from build123d import *

# Parameters (mm, degrees)
SKETCH_1_W          = 15
SKETCH_1_H          = 15
SKETCH_1_R          = 5.5
EXTRUDE_1_DEPTH     = 45
SKETCH_5_W          = 15
SKETCH_5_H          = 15
EXTRUDE_3_DEPTH     = 15
FILLET_2_R          = 7.5
SKETCH_6_R          = 2.1
CUT_EXTRUDE_1_DEPTH = 49.023431781
CUT_EXTRUDE_2_DEPTH = 8
SKETCH_9_W          = 8
SKETCH_9_H          = 8
SKETCH_9_R          = 1.6
EXTRUDE_4_DEPTH     = 7
FILLET_3_R          = 2
SKETCH_11_R         = 3.2
CUT_EXTRUDE_3_DEPTH = 3.75
SKETCH_12_R         = 1.7
CUT_EXTRUDE_4_DEPTH = 10


with BuildPart() as part:
    # ｽｹｯﾁ1 → ﾎﾞｽ - 押し出し1 (new body)
    with BuildSketch(Plane.XY):
        Rectangle(SKETCH_1_W, SKETCH_1_H)
        with Locations(Location((0, 0, 0), (0, 0, 180))):
            Circle(SKETCH_1_R, mode=Mode.SUBTRACT)
    extrude(amount=EXTRUDE_1_DEPTH)

    # ｽｹｯﾁ5 → ﾎﾞｽ - 押し出し3 (add)
    with BuildSketch(Plane.XY.offset(45)):
        Rectangle(SKETCH_5_W, SKETCH_5_H)
    extrude(amount=-EXTRUDE_3_DEPTH)

    # ﾌｨﾚｯﾄ2
    fillet_2_edges = [part.edges().sort_by_distance(p)[0] for p in [
        (0, -7.5, 45),
        (0, 7.5, 45),
    ]]
    fillet(fillet_2_edges, radius=FILLET_2_R - 0.0001)  # a hair under: the kernel refuses the full size

    # ｽｹｯﾁ6 → ｶｯﾄ - 押し出し1 (cut, through all)
    with BuildSketch(Plane(origin=(7.5, 0, 0), x_dir=(0, 0, -1), z_dir=(1, 0, 0))):
        with Locations((-37.5, 0)):
            Circle(SKETCH_6_R)
    extrude(amount=-CUT_EXTRUDE_1_DEPTH, mode=Mode.SUBTRACT)

    # ｽｹｯﾁ7 → ｶｯﾄ - 押し出し2 (cut)
    with BuildSketch(Plane(origin=(7.5, 0, 0), x_dir=(0, 0, -1), z_dir=(1, 0, 0))):
        with BuildLine():
            Line((-37.5, -9.5), (2, -9.5))
            Line((2, -9.5), (2, 9.5))
            Line((2, 9.5), (-37.5, 9.5))
            ThreePointArc((-37.5, 9.5), (-44.217514421, 6.717514421), (-47, 0))
            ThreePointArc((-47, 0), (-44.217514421, -6.717514421), (-37.5, -9.5))
        make_face()
    extrude(amount=-CUT_EXTRUDE_2_DEPTH, mode=Mode.SUBTRACT)

    # ｽｹｯﾁ9 → ﾎﾞｽ - 押し出し4 (add)
    # profile 1 of 4: a face of its own
    with BuildSketch(Plane(origin=(-0.5, 0, 0), x_dir=(0, 0, -1), z_dir=(1, 0, 0))):
        with Locations((-4, -9.477225575)):
            Rectangle(SKETCH_9_W, SKETCH_9_H)
        with Locations((-4, -9.477225575)):
            Circle(SKETCH_9_R, mode=Mode.SUBTRACT)
    # profile 2 of 4: a face of its own
    with BuildSketch(Plane(origin=(-0.5, 0, 0), x_dir=(0, 0, -1), z_dir=(1, 0, 0))):
        with Locations((-26, 9.477225575)):
            Rectangle(SKETCH_9_W, SKETCH_9_H)
        with Locations((-26, 9.477225575)):
            Circle(SKETCH_9_R, mode=Mode.SUBTRACT)
    # profile 3 of 4: a face of its own
    with BuildSketch(Plane(origin=(-0.5, 0, 0), x_dir=(0, 0, -1), z_dir=(1, 0, 0))):
        with Locations((-4, 9.477225575)):
            Rectangle(SKETCH_9_W, SKETCH_9_H)
        with Locations((-4, 9.477225575)):
            Circle(SKETCH_9_R, mode=Mode.SUBTRACT)
    # profile 4 of 4: a face of its own
    with BuildSketch(Plane(origin=(-0.5, 0, 0), x_dir=(0, 0, -1), z_dir=(1, 0, 0))):
        with Locations((-26, -9.477225575)):
            Rectangle(SKETCH_9_W, SKETCH_9_H)
        with Locations((-26, -9.477225575)):
            Circle(SKETCH_9_R, mode=Mode.SUBTRACT)
    extrude(amount=-EXTRUDE_4_DEPTH)

    # ﾌｨﾚｯﾄ3
    fillet_3_edges = [part.edges().sort_by_distance(p)[0] for p in [
        (-4, 13.477225575, 22),
        (-4, 7.5, 30),
        (-4, 13.477225575, 30),
        (-4, 7.5, 22),
        (-4, 13.477225575, 0),
        (-4, 7.5, 8),
        (-4, 13.477225575, 8),
        (-4, -13.477225575, 30),
        (-4, -7.5, 22),
        (-4, -13.477225575, 22),
        (-4, -7.5, 30),
        (-4, -13.477225575, 8),
        (-4, -13.477225575, 0),
        (-4, -7.5, 8),
    ]]
    fillet(fillet_3_edges, radius=FILLET_3_R)

    # ｽｹｯﾁ11 → ｶｯﾄ - 押し出し3 (cut)
    with BuildSketch(Plane.ZY.offset(7.5)):
        with Locations((4, 9.477225575)):
            Circle(SKETCH_11_R)
        with Locations((26, 9.477225575)):
            Circle(SKETCH_11_R)
        with Locations((26, -9.477225575)):
            Circle(SKETCH_11_R)
        with Locations((4, -9.477225575)):
            Circle(SKETCH_11_R)
    extrude(amount=-CUT_EXTRUDE_3_DEPTH, mode=Mode.SUBTRACT)

    # ｽｹｯﾁ12 → ｶｯﾄ - 押し出し4 (cut)
    with BuildSketch(Plane.ZY.offset(7.5)):
        with Locations((15, 0)):
            Circle(SKETCH_12_R)
    extrude(amount=-CUT_EXTRUDE_4_DEPTH, mode=Mode.SUBTRACT)


solid = part.part
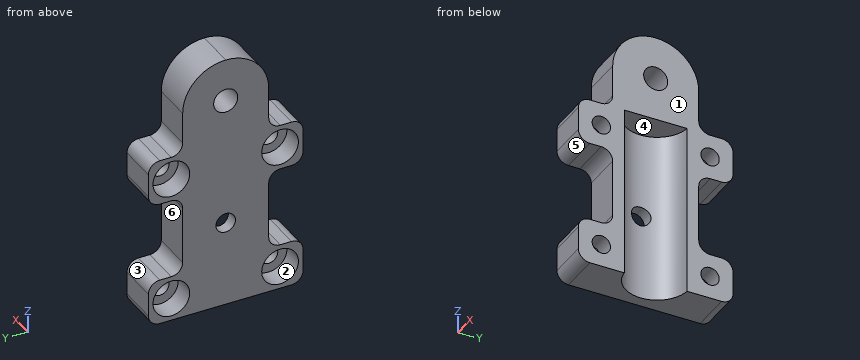
Source: CAD feature listing. Evaluate the final solid. Frame: model axes, mm. Face numbers are marked on the shaded views. A direction names the side the tool comes from. Give positions to 0.01 mm unless a question says otherwise; leave off trailing zeros. Write each loop counter-clockwise with the first axis right and the second up, starting at its lowest first coordinate (ties: lowest second). Pieces come first, ordered by that corner, then holes. Notation, with made-up numbers: M 41,43 L 65,43 A21 cw 65,47 Z; hole C 51,28 d1. An arc over 180 degrees is marked long. Return JSON: item names as keys, results as strings. Group by question number.
1) First-contact query: pin 1 Ø5 at (y, z) = (-9.48, 4) entering from -X; pin 2 Ø2 at (x, z) = (-6.5, 34.5) entering from +Y; pin 3 Ø1.5 at (x, z) = (-6.5, 29) entering from +Y; pin 4 Ø3 at (y, z) = (9.48, 4) entering from +X (1 decimal). Flat tips, straight axial feed; report the tip coordinate or a pass-through.
2) Draft query along Y for the marked faces 1, 2 and 3. Return one class per face: released by +Y, released by -Y, zero draft, split by the parting line, or undercut.
3) Cut plane D-D, the plane y = 12. Output: boundary loops of the cut face in (x, z), then the cut area to 3 significant figures.
4) Ray query, L1, parallel to Y at x = -5.9, z = 4; L2, parallel to Y at x = -1.9, z = 26; L3, parallel to Y at x = -6, z = 37.5. Return the intervals inside material, ascending.
5) Set-up query: the marked faces 4, 5 and 6. Return all of +Z, -Z, +X, -X, +Y, -Y with unobstructed straight access to the full face (end or side cutting, diameter ignored); none if empty.
6) Cut plane C-C, the plane y = 1.25. Output: boundary loops of the cut face in (x, z), then the cut area to 3 significant figures.
7) Cut plane B-B, the plane z = 4. Output: boundary loops of the cut face in (x, y).
8) Cut plane A-A, the plane z = 15. Output: boundary loops of the cut face in (x, y), then the cut area to 3 significant figures.
Data:
{
 "1": {"pin 1": "stops at x = -3.75", "pin 2": "stops at y = 7.5", "pin 3": "stops at y = 13.46", "pin 4": "passes through"},
 "2": {"face 1": "zero draft", "face 2": "undercut", "face 3": "released by +Y"},
 "3": {"outline": "M -7.5,0.07 L -0.5,0.07 L -0.5,7.93 L -7.5,7.93 L -7.5,5.97 L -3.75,5.97 L -3.75,2.03 L -7.5,2.03 Z; M -7.5,22.07 L -0.5,22.07 L -0.5,29.93 L -7.5,29.93 L -7.5,27.97 L -3.75,27.97 L -3.75,24.03 L -7.5,24.03 Z", "area": "80.5 mm²"},
 "4": {"L1": "y = -13.48 to -12.68, -6.28 to 6.28, 12.68 to 13.48", "L2": "y = -13.48 to -11.08, -7.88 to -5.16, 5.16 to 7.88, 11.08 to 13.48", "L3": "y = -7.5 to -2.1, 2.1 to 7.5"},
 "5": {"face 4": "-Z, +X", "face 5": "+X, -X, -Y", "face 6": "+X, -X, +Y"},
 "6": {"outline": "M -7.5,0 L -5.36,0 L -5.36,13.85 L -7.5,13.85 Z; M -7.5,16.15 L -5.36,16.15 L -5.36,30 L -0.5,30 L -0.5,35.81 L -7.5,35.81 Z; M -7.5,39.19 L -0.5,39.19 L -0.5,44.9 L -7.5,44.9 Z", "area": "140 mm²"},
 "7": {"outline": "M -7.5,-13.48 L -0.5,-13.48 L -0.5,-11.08 L -3.75,-11.08 L -3.75,-12.68 L -7.5,-12.68 Z; M -7.5,-6.28 L -3.75,-6.28 L -3.75,-7.88 L -0.5,-7.88 L -0.5,-5.48 A5.5 cw -0.5,5.48 L -0.5,7.88 L -3.75,7.88 L -3.75,6.28 L -7.5,6.28 Z; M -7.5,12.68 L -3.75,12.68 L -3.75,11.08 L -0.5,11.08 L -0.5,13.48 L -7.5,13.48 Z"},
 "8": {"outline": "M -7.5,-7.5 L -0.5,-7.5 L -0.5,-5.48 A5.5 cw -5.23,-1.7 L -7.5,-1.7 Z; M -7.5,1.7 L -5.23,1.7 A5.5 cw -0.5,5.48 L -0.5,7.5 L -7.5,7.5 Z", "area": "55.9 mm²"}
}
